Autodesk Inventor part; units mm, degrees
ref_plane "Work Plane1" through (-31, -15, -1.6) normal (0, 0, -1) x (0, 1, 0)
ref_plane "YZ Plane" through (0, 0, 0) normal (1, 0, 0) x (0, 1, 0)
ref_plane "XZ Plane" through (0, 0, 0) normal (0, 1, 0) x (-1, 0, 0)
sketch "Sketch1" plane through (0, 0, 0) normal (0, 0, 1) x (1, 0, 0)
  circle A0 centre (28, -12) radius 1.6 construction
  circle A1 centre (-25, -0.5) radius 1.6 construction
  circle A2 centre (28, 12) radius 1.6 construction
  line L0 (-28, -15) -> (28, -15)
  line L1 (-31, 12) -> (-31, -12)
  line L2 (28, 15) -> (-28, 15)
  line L3 (31, -12) -> (31, 12)
  circle A3 centre (28, -12) radius 3
  circle A4 centre (28, 12) radius 3
  circle A5 centre (-25, -0.5) radius 3
  circle A6 centre (28, -12) radius 1.4
  circle A7 centre (28, 12) radius 1.4
  circle A8 centre (-25, -0.5) radius 1.4
  point P0 (0, 0)
extrude "Extrusion1" add sketch "Sketch1" along normal blind 3
sketch "Sketch2" plane through (28, -12, 3) normal (0, 0, 1) x (1, 0, 0)
  line L0 (-59, 24) -> (-59, 0)
  line L1 (0, 27) -> (-56, 27)
  line L2 (-56, -3) -> (0, -3)
  line L3 (3, 0) -> (3, 24)
  line L4 (-59, 27) -> (3, 27)
  line L5 (3, 27) -> (3, -3)
  line L6 (3, -3) -> (-59, -3)
  line L7 (-59, -3) -> (-59, 27)
  point P0 (-28, 12)
extrude "Extrusion2" add sketch "Sketch2" along normal blind 2
fillet "Fillet1" radius 3 4 edges at (31, -15, 4) (31, 15, 4) (-31, 15, 4) (-31, -15, 4)
sketch "Sketch3" plane through (28, -12, 5) normal (0, 0, 1) x (1, 0, 0)
  arc A0 (-59, 0) -> (-56, -3) centre (-56, 0) ccw
  line L0 (-56, -3) -> (0, -3)
  arc A1 (0, -3) -> (3, 0) centre (0, 0) ccw
  line L1 (3, 0) -> (3, 24)
  arc A2 (3, 24) -> (0, 27) centre (0, 24) ccw
  line L2 (0, 27) -> (-56, 27)
  arc A3 (-56, 27) -> (-59, 24) centre (-56, 24) ccw
  line L3 (-59, 24) -> (-59, 0)
  line L4 (5.5, 24) -> (5.5, 0)
  arc A4 (0, -5.5) -> (5.5, 0) centre (0, 0) ccw
  line L5 (0, -5.5) -> (-56, -5.5)
  arc A5 (-61.5, 0) -> (-56, -5.5) centre (-56, 0) ccw
  line L6 (-61.5, 0) -> (-61.5, 24)
  arc A6 (-56, 29.5) -> (-61.5, 24) centre (-56, 24) ccw
  line L7 (-56, 29.5) -> (0, 29.5)
  arc A7 (5.5, 24) -> (0, 29.5) centre (0, 24) ccw
  point P0 (-28, 12)
  dimension "d9" = 2.5
ref_plane "Work Plane1" through (-31, -15, -1.6) normal (0, 0, -1) x (0, 1, 0)
extrude "Extrusion3" add sketch "Sketch3" against normal up to surface (6.6 mm away)
sketch "Sketch4" plane through (28, 17.5, -1.6) normal (0, 0, -1) x (-1, 0, 0)
  arc A0 (59, -5.5) -> (56, -2.5) centre (56, -5.5) ccw
  line L0 (59, -29.5) -> (59, -5.5)
  arc A1 (56, -32.5) -> (59, -29.5) centre (56, -29.5) ccw
  line L1 (0, -32.5) -> (56, -32.5)
  arc A2 (-3, -29.5) -> (0, -32.5) centre (0, -29.5) ccw
  line L2 (-3, -5.5) -> (-3, -29.5)
  arc A3 (0, -2.5) -> (-3, -5.5) centre (0, -5.5) ccw
  line L3 (56, -2.5) -> (0, -2.5)
  arc A4 (56, -35) -> (61.5, -29.5) centre (56, -29.5) ccw
  line L4 (61.5, -5.5) -> (61.5, -29.5)
  arc A5 (61.5, -5.5) -> (56, 0) centre (56, -5.5) ccw
  line L5 (0, 0) -> (56, 0)
  arc A6 (0, 0) -> (-5.5, -5.5) centre (0, -5.5) ccw
  line L6 (-5.5, -29.5) -> (-5.5, -5.5)
  arc A7 (-5.5, -29.5) -> (0, -35) centre (0, -29.5) ccw
  line L7 (56, -35) -> (0, -35)
  arc A8 (0, -2) -> (-3.5, -5.5) centre (0, -5.5) ccw
  line L8 (-3.5, -5.5) -> (-3.5, -29.5)
  arc A9 (-3.5, -29.5) -> (0, -33) centre (0, -29.5) ccw
  line L9 (0, -33) -> (56, -33)
  arc A10 (56, -33) -> (59.5, -29.5) centre (56, -29.5) ccw
  line L10 (59.5, -29.5) -> (59.5, -5.5)
  arc A11 (59.5, -5.5) -> (56, -2) centre (56, -5.5) ccw
  line L11 (56, -2) -> (0, -2)
  point P0 (28, -17.5)
  dimension "d12" = 0.5
extrude "Extrusion4" cut sketch "Sketch4" against normal up to surface (1.6 mm away) contours L11 A11 L10 A10 L9 A9 L8 A8
sketch "Sketch5" plane through (33.5, -12, 5) normal (1, 0, 0) x (0, 0, -1)
  line L0 (6.6, 20.7422) -> (10.115, 20.7422)
  line L1 (10.115, 5.7422) -> (6.6, 5.7422)
  line L2 (6.6, 20.7422) -> (4.1, 20.7422)
  line L3 (4.1, 20.7422) -> (4.1, 5.7422)
  line L4 (4.1, 5.7422) -> (6.6, 5.7422)
  line L5 (6.6, 5.7422) -> (6.6, 20.7422)
  point P0 (5, 12)
  dimension "d15" = 2.5
extrude "Extrusion5" cut sketch "Sketch5" against normal blind 21.75
fillet "Fillet2" radius 2 2 edges at (32.25, 8.7422, 0.9) (32.25, -6.2578, 0.9)
fillet "Fillet3" radius 2 4 edges at (31, 12, 1.5) (28, 15, 1.5) (28, -15, 1.5) (31, -12, 1.5)
fillet "Fillet4" radius 2 1 edges at (-28, -0.5, 3)
properties part number "case_base"
Input: part model. Units: mm. Frame: model coordinates. A direction names the side the tool comes from. Coordinates: 2 decimals unless noted, no trailing zeros. Write each loop counter-clockwise with the first axis right and the second up, starting at its lowest first coordinate (ties: lowest second). Pieces come first, ordered by that corner, then holes. Notation, with made-up numbers: (-35, 1) -> (-25, 1) arc R32 cw to (-25, 36) -> close; hole circle Ø7 at (21, 33). An arc over 180 degrees is marked (long way). Write each question's results on one line, items separated by ' | '.
Item 1: Section query C-C on x = -25. Return loops of the section in (y, z).
Conclusion:
outline: (-17.5, -1.6) -> (-15.5, -1.6) -> (-15.5, 0) -> (-15, 0) -> (-15, 3) -> (-5.5, 3) arc R2 cw to (-3.5, 1) -> (-3.5, 0) -> (-1.9, 0) -> (-1.9, 3) -> (0.9, 3) -> (0.9, 0) -> (2.5, 0) -> (2.5, 1) arc R2 cw to (4.5, 3) -> (15, 3) -> (15, 0) -> (15.5, 0) -> (15.5, -1.6) -> (17.5, -1.6) -> (17.5, 5) -> (-17.5, 5) -> close
Item 2: Material intervals for probe 1 along Y at (x, z) = (-25, 1); probe 2 along Y at (x, z) = (5.5, 2.5); probe 3 along Y at (x, z) = (28, 1.25), sorted ascending.
Conclusion:
probe 1: y = -17.5 to -15, -3.5 to -1.9, 0.9 to 2.5, 15 to 17.5 | probe 2: y = -17.5 to -15, 15 to 17.5 | probe 3: y = -17.5 to -13.4, -10.6 to -9, 9 to 10.6, 13.4 to 17.5
Item 3: Mould query, pull axis Y, two halves, no side actions, for faces 4 (the flat face through (-33.5, 0, 2)), 5 (the cylindrical face through (26.97, 11.05, 1.48)), 6 (the cylindrical face through (-31.85, 15.93, 1.75)). Classes: +Y half, -Y half, draft (parallel to the pull), parting line (faces both ways), or undercut.
Conclusion:
face 4: draft | face 5: undercut | face 6: +Y half
Item 4: Section query A-A on y = -0.5. Return loops of the section in (x, z), plus the area to 3 significant figures.
Conclusion:
outline: (-33.5, -1.6) -> (-31.5, -1.6) -> (-31.5, 0) -> (-31, 0) -> (-31, 3) -> (-30, 3) arc R2 cw to (-28, 1) -> (-28, 0) -> (-26.4, 0) -> (-26.4, 3) -> (-23.6, 3) -> (-23.6, 0) -> (-22, 0) -> (-22, 1) arc R2 cw to (-20, 3) -> (31, 3) -> (31, 0.9) -> (33.5, 0.9) -> (33.5, 5) -> (-33.5, 5) -> close | area: 161 mm^2
Item 5: Pin query (flat end, axial travel): pin 1 Ø1 at (y, z) = (-13.5, -0.5) entering from +X; pin 2 Ø0.8 at (y, z) = (-4.5, -1) entering from +X; pin 3 Ø15.5 at (x, y) = (15.5, -7.5) entering from -Z. Return the tip coordinate at first contact, or that it passes through.
Conclusion:
pin 1: stops at x = 33.41 | pin 2: stops at x = -31.5 | pin 3: stops at z = 0
Item 6: Section query B-B on x = -14. Return loops of the section in (y, z).
Conclusion:
outline: (-17.5, -1.6) -> (-15.5, -1.6) -> (-15.5, 0) -> (-15, 0) -> (-15, 3) -> (15, 3) -> (15, 0) -> (15.5, 0) -> (15.5, -1.6) -> (17.5, -1.6) -> (17.5, 5) -> (-17.5, 5) -> close
Item 7: Set-up query: faces 1 (the cylindrical face through (31.85, -15.93, 1.75)), 2 (the cylindrical face through (32.268, -5.656, 0.33)), 3 (the flat face through (0, 0, 3)). Return all of +Z, -Z, +X, -X, +Y, -Y with unobstructed straight access to the full face (end or side cutting, diameter ignored); none if empty.
Conclusion:
face 1: +Z, -Z, +X, -Y | face 2: -Z, +X | face 3: -Z
